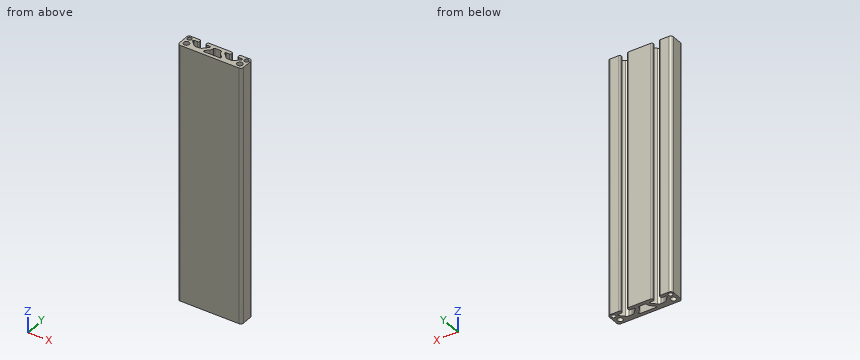
Autodesk Inventor part; units mm, degrees
ref_plane "YZ Plane" through (0, 0, 0) normal (1, 0, 0) x (0, 1, 0)
ref_plane "XZ Plane" through (0, 0, 0) normal (0, 1, 0) x (-1, 0, 0)
ref_plane "XY Plane" through (0, 0, 0) normal (0, 0, 1) x (1, 0, 0)
sketch "Sketch1" plane through (0, 0, 0) normal (0, 0, 1) x (1, 0, 0)
  circle A0 centre (31.75, -3.175) radius 3.3274
  circle A1 centre (33.8988, 5.2764) radius 2.5527
  circle A2 centre (-33.8988, 5.2764) radius 2.5527
  circle A3 centre (-31.75, -3.175) radius 3.3274
  line L0 (-9.5899, -5.461) -> (9.5899, -5.461)
  arc A4 (-10.4789, -4.572) -> (-9.5899, -5.461) centre (-9.5899, -4.572) ccw
  line L1 (-10.4789, -4.1197) -> (-10.4789, -4.572)
  arc A5 (-10.2185, -3.4911) -> (-10.4789, -4.1197) centre (-9.5899, -4.1197) ccw
  line L2 (-6.264, 0.4634) -> (-10.2185, -3.4911)
  arc A6 (-6.264, 0.4634) -> (-4.8728, 3.822) centre (-9.6226, 3.822) ccw
  line L3 (-4.8728, 4.191) -> (-4.8728, 3.822)
  arc A7 (-3.6028, 5.461) -> (-4.8728, 4.191) centre (-3.6028, 4.191) ccw
  line L4 (3.6028, 5.461) -> (-3.6028, 5.461)
  arc A8 (4.8728, 4.191) -> (3.6028, 5.461) centre (3.6028, 4.191) ccw
  line L5 (4.8728, 3.822) -> (4.8728, 4.191)
  arc A9 (4.8728, 3.822) -> (6.264, 0.4634) centre (9.6226, 3.822) ccw
  line L6 (10.2185, -3.4911) -> (6.264, 0.4634)
  arc A10 (10.4789, -4.1197) -> (10.2185, -3.4911) centre (9.5899, -4.1197) ccw
  line L7 (10.4789, -4.572) -> (10.4789, -4.1197)
  arc A11 (9.5899, -5.461) -> (10.4789, -4.572) centre (9.5899, -4.572) ccw
  arc A12 (24.638, 9.525) -> (23.114, 8.001) centre (24.638, 8.001) ccw
  line L8 (23.114, 8.001) -> (23.114, 6.731)
  arc A13 (23.114, 6.731) -> (24.384, 5.461) centre (24.384, 6.731) ccw
  line L9 (24.384, 5.461) -> (28.448, 5.461)
  arc A14 (29.337, 4.572) -> (28.448, 5.461) centre (28.448, 4.572) ccw
  line L10 (29.337, 4.572) -> (29.337, 4.2554)
  arc A15 (29.0766, 3.6267) -> (29.337, 4.2554) centre (28.448, 4.2554) ccw
  line L11 (29.0766, 3.6267) -> (24.1741, -1.2758)
  arc A16 (20.8154, -2.667) -> (24.1741, -1.2758) centre (20.8154, 2.0828) ccw
  line L12 (20.8154, -2.667) -> (17.2846, -2.667)
  arc A17 (13.9259, -1.2758) -> (17.2846, -2.667) centre (17.2846, 2.0828) ccw
  line L13 (13.9259, -1.2758) -> (9.0234, 3.6267)
  arc A18 (8.763, 4.2554) -> (9.0234, 3.6267) centre (9.652, 4.2554) ccw
  line L14 (8.763, 4.2554) -> (8.763, 4.572)
  arc A19 (9.652, 5.461) -> (8.763, 4.572) centre (9.652, 4.572) ccw
  line L15 (9.652, 5.461) -> (13.716, 5.461)
  arc A20 (13.716, 5.461) -> (14.986, 6.731) centre (13.716, 6.731) ccw
  line L16 (14.986, 6.731) -> (14.986, 8.001)
  arc A21 (14.986, 8.001) -> (13.462, 9.525) centre (13.462, 8.001) ccw
  line L17 (13.462, 9.525) -> (-13.462, 9.525)
  arc A22 (-13.462, 9.525) -> (-14.986, 8.001) centre (-13.462, 8.001) ccw
  line L18 (-14.986, 8.001) -> (-14.986, 6.731)
  arc A23 (-14.986, 6.731) -> (-13.716, 5.461) centre (-13.716, 6.731) ccw
  line L19 (-13.716, 5.461) -> (-9.652, 5.461)
  arc A24 (-8.763, 4.572) -> (-9.652, 5.461) centre (-9.652, 4.572) ccw
  line L20 (-8.763, 4.572) -> (-8.763, 4.2554)
  arc A25 (-9.0234, 3.6267) -> (-8.763, 4.2554) centre (-9.652, 4.2554) ccw
  line L21 (-9.0234, 3.6267) -> (-13.9259, -1.2758)
  arc A26 (-17.2846, -2.667) -> (-13.9259, -1.2758) centre (-17.2846, 2.0828) ccw
  line L22 (-17.2846, -2.667) -> (-20.8154, -2.667)
  arc A27 (-24.1741, -1.2758) -> (-20.8154, -2.667) centre (-20.8154, 2.0828) ccw
  line L23 (-24.1741, -1.2758) -> (-29.0766, 3.6267)
  arc A28 (-29.337, 4.2554) -> (-29.0766, 3.6267) centre (-28.448, 4.2554) ccw
  line L24 (-29.337, 4.2554) -> (-29.337, 4.572)
  arc A29 (-28.448, 5.461) -> (-29.337, 4.572) centre (-28.448, 4.572) ccw
  line L25 (-28.448, 5.461) -> (-24.384, 5.461)
  arc A30 (-24.384, 5.461) -> (-23.114, 6.731) centre (-24.384, 6.731) ccw
  line L26 (-23.114, 6.731) -> (-23.114, 8.001)
  arc A31 (-23.114, 8.001) -> (-24.638, 9.525) centre (-24.638, 8.001) ccw
  line L27 (-24.638, 9.525) -> (-34.925, 9.525)
  arc A32 (-34.925, 9.525) -> (-38.1, 6.35) centre (-34.925, 6.35) ccw
  line L28 (-38.1, 6.35) -> (-38.1, -6.35)
  arc A33 (-38.1, -6.35) -> (-34.925, -9.525) centre (-34.925, -6.35) ccw
  line L29 (-34.925, -9.525) -> (34.925, -9.525)
  arc A34 (34.925, -9.525) -> (38.1, -6.35) centre (34.925, -6.35) ccw
  line L30 (38.1, -6.35) -> (38.1, 6.35)
  arc A35 (38.1, 6.35) -> (34.925, 9.525) centre (34.925, 6.35) ccw
  line L31 (34.925, 9.525) -> (24.638, 9.525)
  point P0 (0, 0)
extrude "Extrusion1" add sketch "Sketch1" against normal blind 304.8
properties part number "3075"
CAD build for the part. Positions are in the model's coordinates, mm. Round coordinates to 2 decimals unless told otherwise and drop trailing zeros.
Item 1: Pin check, flat tips, straight feed: pin 1 (5.5 mm diameter, centred on x = -31.75, y = -3.175, fed in from -Z); pin 2 (1.1 mm diameter, centred on x = 18.5, z = -170, fed in from +Y); pin 3 (0.6 mm diameter, centred on y = 7.5, z = -133, fed in from +X); pin 4 (1.4 mm diameter, centred on y = 7.5, z = -152.5, fed in from +X). Stop position of each tip, or through.
Item 2: Saw through at A-A on z = -97. State how many separate pieces and enclosed holes the cut face has, then the cut area to 3 significant figures.
Item 3: Probe line 1 along X through (y, z) = (6, -160); line 2 along Y through (x, z) = (3.5, -52) (3 decimals); line 3 along X through (y, z) = (-3, -117.5). List the from-to ranges inside material, lowest first.
Reported:
1. pin 1: passes through
1. pin 2: stops at y = -2.67
1. pin 3: stops at x = 37.98
1. pin 4: stops at x = 38.07
2. separate pieces: 1
2. enclosed holes: 5
2. area: 860 mm2
3. line 1: x = -38.1 to -36.35, -31.45 to -23.35, -14.75 to 14.75, 23.35 to 31.45, 36.35 to 38.1
3. line 2: y = -9.525 to -5.461, 5.461 to 9.525
3. line 3: x = -38.1 to -35.07, -28.43 to -9.73, 9.73 to 28.43, 35.07 to 38.1
